The listing builds one solid part. Answer for the finished solid, in the listing's coordinates (mm). A direction names the side the tool comes from. Coordinates: 2 decimals unless noted, no trailing zeros. Order: outer loops, then holes, each group sorted by start corner. A loop starts at its lowest first (then second) coordinate and runs counter-clockwise, first axis right, second up. Notation, with made-up numbers: (-16, -34.5) -> (25, -34.5) arc R23 cw to (25, -2.5) -> close; hole circle Ø3 at (-12.75, 55.5). An arc over 180 degrees is marked (long way). Answer in a Markdown table with one row per item.
```python
from build123d import *

# Parameters (mm, degrees)
BOSS_EXTRU_1_DEPTH      = 210
ENL_V_MAT_EXTRU_4_DEPTH = 922.018231875
ENL_V_MAT_EXTRU_5_DEPTH = 922.018231875
ENL_V_MAT_EXTRU_6_DEPTH = 923.94578116
ENL_V_MAT_EXTRU_7_DEPTH = 5
CHANFREIN1_SIZE         = 5


with BuildPart() as part:
    # Esquisse1 → Boss.-Extru.1 (new body)
    with BuildSketch(Plane.XY):
        Polygon((0, 0), (0, 815), (-374.098360656, 815), align=None)
    extrude(amount=-BOSS_EXTRU_1_DEPTH)

    # Esquisse4 → Enlèv. mat.-Extru.4 (cut, through all)
    with BuildSketch(Plane(origin=(0, 815, 0), x_dir=(1, 0, 0), z_dir=(0, 1, 0))):
        Polygon((-40, 210), (-374.098360656, 0), (-374.098360656, 210), align=None)
    extrude(amount=-ENL_V_MAT_EXTRU_4_DEPTH, mode=Mode.SUBTRACT)

    # Esquisse5 → Enlèv. mat.-Extru.5 (cut, through all)
    with BuildSketch(Plane(origin=(0, 0, 0), x_dir=(-0.8560075896570557, 0.14330783348955523, 0.49670300110835625), z_dir=(-0.5169632544480486, -0.23729460859910434, -0.8224598849064191))):
        Polygon((437.026920294, 783.059419447), (0, 0), (-104.307630233, 58.214282686), (12.488254061, 841.273702133), (46.728557648, 841.273702133), align=None)
    extrude(amount=ENL_V_MAT_EXTRU_5_DEPTH, mode=Mode.SUBTRACT)

    # Esquisse6 → Enlèv. mat.-Extru.6 (cut, through all)
    with BuildSketch(Plane(origin=(5.169632544, 2.372946086, 8.224598849), x_dir=(-0.8560075896570557, 0.14330783348955523, 0.49670300110835625), z_dir=(-0.5169632544480486, -0.23729460859910434, -0.8224598849064191))):
        Polygon((437.026920294, 783.059419447), (46.728557648, 841.273702133), (12.488254061, 841.273702133), (0, 757.546051675), (0, 0), align=None)
    extrude(amount=-ENL_V_MAT_EXTRU_6_DEPTH, mode=Mode.SUBTRACT)

    # Esquisse7 → Enlèv. mat.-Extru.7 (cut)
    with BuildSketch(Plane(origin=(5.169632544, 2.372946086, 8.224598849), x_dir=(0.8560075896570555, -0.14330783348955536, -0.4967030011083565), z_dir=(0.5169632544480489, 0.23729460859910445, 0.8224598849064189))):
        Polygon((-45.786058342, 173.266527892), (-36.039236809, 175.802293869), (-36.039236809, 790.231286712), (-46.25858999, 808.542197087), (-323.672371858, 767.165020382), (-348.758261389, 716.128366398), align=None)
    extrude(amount=-ENL_V_MAT_EXTRU_7_DEPTH, mode=Mode.SUBTRACT)

    # Chanfrein1
    chanfrein1_edges = [part.edges().sort_by_distance(p)[0] for p in [
        (-32.436720565, 174.743826797, -23.949101615),
        (-166.281649801, 456.726474452, -21.176992916),
        (-285.218046516, 761.94965633, -34.481068848),
        (-155.747039223, 784.670394973, -122.416375357),
        (-32.638965904, 775.141493599, -197.047605933),
        (-28.265043962, 470.438107301, -111.884408124),
    ]]
    chamfer(chanfrein1_edges, length=CHANFREIN1_SIZE - 0.0001)  # a hair under: the kernel refuses the full size


solid = part.part
```
(1) Flat-ended cylindrical pins translate along their axes: pin 1 (3 mm diameter, centred on x = -67, y = 472, fed in from +Z); pin 2 (8 mm diameter, centred on x = -233, y = 605, fed in from -Z); pin 3 (1.5 mm diameter, centred on y = 295.5, z = -72, fed in from -X). Find the tip coordinate at first contact, or state that the pin passes through.
Check values:
| item | result |
|---|---|
| pin 1 | z = -86.95 |
| pin 2 | z = -30.87 |
| pin 3 | x = -22.33 |
(2) For a pull along X with two mould halves and no side action, classify faces 1 (the flat face through (0, 383, -105)), 2 (the flat face through (-29.161, 467.254, -107.406)), 3 (the flat face through (-106.535, 517.457, -82.332)), 4 (the flat face through (-197, 815, -105)) as released by +X, released by -X, zero draft, split by the parting line, or undercut.
Check values:
| item | result |
|---|---|
| face 1 | released by +X |
| face 2 | undercut |
| face 3 | released by -X |
| face 4 | zero draft |
(3) Find the intervals of material crossed by line 1 along Z through (x, y) = (-162, 657); line 2 along X through (y, z) = (726.5, -72.5); line 3 along X through (y, z) = (150.5, -18), in increasing order. Write a range as from..to.
Check values:
| item | result |
|---|---|
| line 1 | -87.73..-81.65 |
| line 2 | -218.13..-208.46 |
| line 3 | -40.44..-21.1 |
(4) A cutting plane is placed at D-D, the plane y = 124.5. Determine the outline of the cut face in (x, z), then the cut area to 3 significant figures.
Check values:
| item | result |
|---|---|
| outline | (-57.15, 0) -> (0, -35.92) -> (0, -23.76) -> (-37.8, 0) -> close |
| area | 577 mm² |
(5) A cutting plane is placed at C-C, the plane x = -307. Determine the outline of the cut face in (y, z), then the cut area to 3 significant figures.
Check values:
| item | result |
|---|---|
| outline | (668.82, 0) -> (815, -42.18) -> (815, -30.02) -> (710.96, 0) -> close |
| area | 1,520 mm² |
(6) Which of the six approach directions +Z, -Z, +X, -X, +Y, -Y give full straight-line access (tool end or side, diameter ignored) to faces 5 (the flat face through (-188, 440, 0)), 6 (the flat face through (-152.49, 782.793, -120.925))?
Check values:
| item | result |
|---|---|
| face 5 | +Z, +X, -X, +Y, -Y |
| face 6 | +Z, +X |
